Part print with two shaded views. Sizes in mm from the minimum x, y, z corner. Give positions to 0.01 mm unless a question says otherwise; leave off trailing zeros. Order: outer loops, then holes, each group sorted by start corner. A loop starts at its lowest first (then second) coordinate and runs counter-clockwise, first axis right, second up. Notation, with made-up numbers: M 88,75.5 L 121,75.5 A17 ccw 121,100.5 Z; hole C 87.5,30.5 d3. An arc over 180 degrees is marked long. Return JSON: item names as keys, results as strings. Group by question number.
1. Slice it at C-C on z = 14.5. List the corners of the cut face in (x, y) (3 decimals), then the cut area to 3 significant figures.
2. Slice it at A-A on x = 58. List the corners of the cut face in (y, z), then the cut area to 3 significant figures.
3. Wall check: probe 1 along Y at (x, z) = (37, 20.5); probe 2 along X at (y, z) = (7.5, 18); probe 3 along Y at (x, z) = (81.5, 2). Give the ranges that are in metal, low to high. Write a range as [from, to].
4. Two-plate mould, pull along Y, no slides. Class the marked faces 1, 2 and 3: released by +Y, released by -Y, zero draft, split by the parting line, or undercut.
5. Slice it at B-B on y = 10.5. List the corners of the cut face in (x, z).
6. Pin check, flat tips, straight feed: pin 1 (2 mm diameter, centred on y = 5, z = 14.5, fed in from -X); pin 2 (1.5 mm diameter, centred on y = 9, z = 4, fed in from -X). Stop position of each tip, or through.
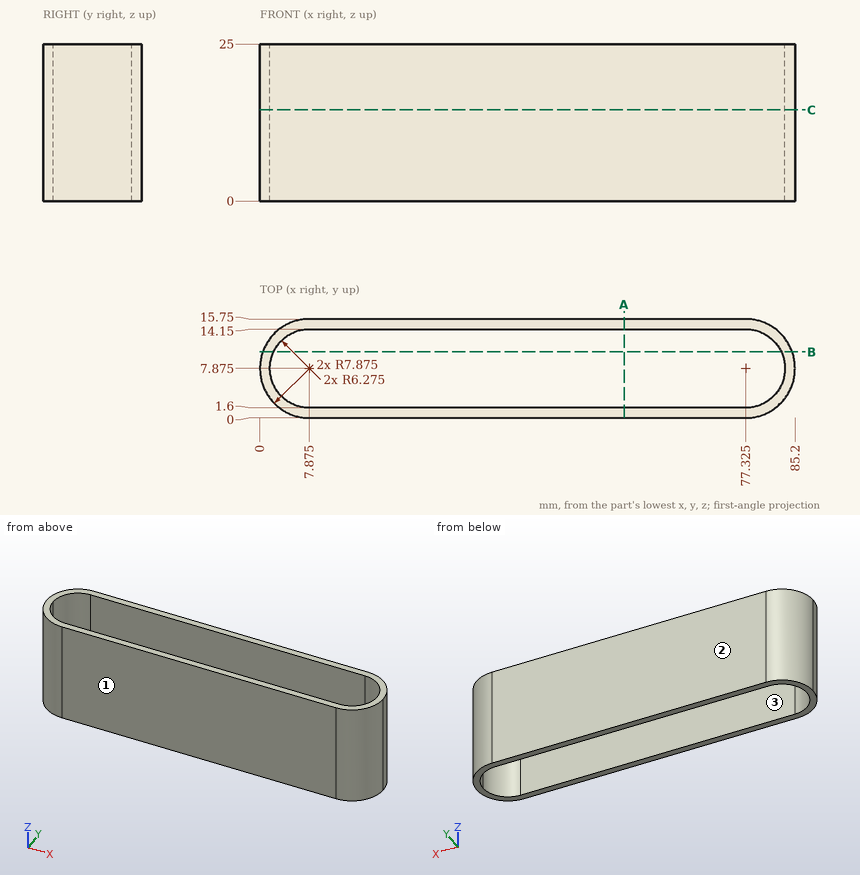
Result:
{
 "1": {"outline": "M 7.875,0 L 77.325,0 A7.875 ccw 77.325,15.75 L 7.875,15.75 A7.875 ccw Z; hole M 7.875,1.6 L 77.325,1.6 A6.275 ccw 77.325,14.15 L 7.875,14.15 A6.275 ccw Z", "area": "293 mm2"},
 "2": {"outline": "M 0,0 L 1.6,0 L 1.6,25 L 0,25 Z; M 14.15,0 L 15.75,0 L 15.75,25 L 14.15,25 Z", "area": "80.0 mm2"},
 "3": {"probe 1": "y = [0, 1.6], [14.15, 15.75]", "probe 2": "x = [0.01, 1.61], [83.59, 85.19]", "probe 3": "y = [1.2, 3.19], [12.56, 14.55]"},
 "4": {"face 1": "released by -Y", "face 2": "released by +Y", "face 3": "undercut"},
 "5": {"outline": "M 0.45,0 L 2.18,0 L 2.18,25 L 0.45,25 Z; M 83.02,0 L 84.75,0 L 84.75,25 L 83.02,25 Z"},
 "6": {"pin 1": "stops at x = 0.23", "pin 2": "stops at x = 0.01"}
}
